For this review, take the finished solid that the model builds, in its own axes (mm). Face numbers are marked on the shaded views. A direction names the side the tool comes from. Give positions to 0.01 mm unless a question says otherwise; leave off trailing zeros. Loops run counter-clockwise (first coordinate to the right, second up) from the corner with the lowest first, then second, coordinate; pieces in that order, holes last. Notation, with made-up numbers: (37.5, 66) -> (71.5, 66) arc R20 ccw to (71.5, 85) -> close; hole circle Ø8 at (88, 13). An arc over 180 degrees is marked (long way). Answer as CSV lines item,"result". Start each with the question number.
Item 1: For L1, parallel to X at y = 6.75, z = -5.25; L2, parallel to Y at x = 1.25, z = -4.25, list the stretches that pass through material, from the lowest coordinate up. Write a range as from..to.
Item 2: The part is to be moulded in two halves that separate along Z. For the marked faces 1, 2 and 3, say which applies: +Z half, -Z half, draft (parallel to the pull), parting line (faces both ways), or undercut.
Item 3: Add section D-D on y = 10.25. State the section outline as (x, z) points, plus the area to 3 significant figures.
Item 4: Add section C-C on x = 1. State the section outline as (y, z) points, plus the area to 3 significant figures.
Item 5: Add section A-A on y = 2.75. State the section outline as (x, z) points.
Item 6: Clearance check with flat-ended pins moving along their axes: P1, Ø1, axis at x = -0.5, z = 2.5, coming from the +Y side; P2, Ø7.5, axis at x = -3.5, z = -2, coming from the +Y side. State where each tip first meets the part, or that it passes through.
Item 7: Machinability: for the marked faces 4 and 5, which of the approach directions +Z, -Z, +X, -X, +Y, -Y give a long, thin tool a straight path to every point of the face, cutting with its end or side? Answer none if there is none.
Item 8: Add section B-B on z = 1.5. State the section outline as (x, y) points, plus the area to 3 significant figures.
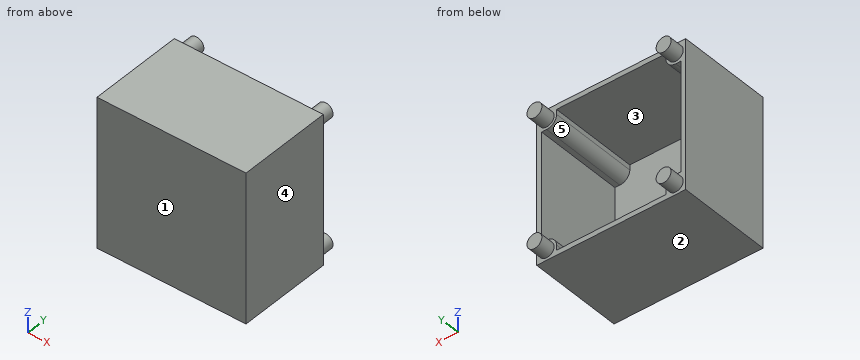
```python
from build123d import *

# Parameters (mm, degrees)
SKETCH_1_W          = 15
SKETCH_1_H          = 15
EXTRUDE_1_DEPTH     = 9.5
CUT_EXTRUDE_1_DEPTH = 9
SKETCH_5_R          = 0.75
EXTRUDE_2_DEPTH     = 1.5


with BuildPart() as part:
    # 草图1 → 凸台-拉伸1 (new body)
    with BuildSketch(Plane(origin=(0, 0, 0), x_dir=(1, 0, 0), z_dir=(0, 1, 0))):
        Rectangle(SKETCH_1_W, SKETCH_1_H)
    extrude(amount=EXTRUDE_1_DEPTH)

    # 草图2 → 切除-拉伸1 (cut)
    with BuildSketch(Plane(origin=(0, 9.5, 0), x_dir=(-1, 0, 0), z_dir=(0, 1, 0))):
        with BuildLine():
            Line((6.5, -5.5), (7, -5.5))
            Line((7, -5.5), (7, 5.5))
            Line((7, 5.5), (6.5, 5.5))
            ThreePointArc((6.5, 5.5), (5.792893219, 5.792893219), (5.5, 6.5))
            Line((5.5, 6.5), (5.5, 7))
            Line((5.5, 7), (-5.5, 7))
            Line((-5.5, 7), (-5.5, 6.5))
            ThreePointArc((-5.5, 6.5), (-5.792893219, 5.792893219), (-6.5, 5.5))
            Line((-6.5, 5.5), (-7, 5.5))
            Line((-7, 5.5), (-7, -5.5))
            Line((-7, -5.5), (-6.5, -5.5))
            ThreePointArc((-6.5, -5.5), (-5.792893219, -5.792893219), (-5.5, -6.5))
            Line((-5.5, -6.5), (-5.5, -7))
            Line((-5.5, -7), (5.5, -7))
            Line((5.5, -7), (5.5, -6.5))
            ThreePointArc((5.5, -6.5), (5.792893219, -5.792893219), (6.5, -5.5))
        make_face()
    extrude(amount=-CUT_EXTRUDE_1_DEPTH, mode=Mode.SUBTRACT)

    # 草图5 → 凸台-拉伸2 (add)
    with BuildSketch(Plane(origin=(0, 9.5, 0), x_dir=(-1, 0, 0), z_dir=(0, 1, 0))):
        with Locations(Location((6.5, -6.5, 0), (0, 0, 270))):
            Circle(SKETCH_5_R)
        with Locations(Location((6.5, 6.5, 0), (0, 0, 270))):
            Circle(SKETCH_5_R)
        with Locations(Location((-6.5, 6.5, 0), (0, 0, 270))):
            Circle(SKETCH_5_R)
        with Locations(Location((-6.5, -6.5, 0), (0, 0, 270))):
            Circle(SKETCH_5_R)
    extrude(amount=EXTRUDE_2_DEPTH)


solid = part.part
```
Computed values:
1,L1,"-7.5..-7, 7..7.5"
1,L2,"0..0.5"
2,face 1,"draft"
2,face 2,"-Z half"
2,face 3,"undercut"
3,outline,"circle Ø1.5 at (-6.5, -6.5); circle Ø1.5 at (-6.5, 6.5); circle Ø1.5 at (6.5, -6.5); circle Ø1.5 at (6.5, 6.5)"
3,area,"7.07 mm²"
4,outline,"(0, -7.5) -> (9.5, -7.5) -> (9.5, -7) -> (0.5, -7) -> (0.5, 7) -> (9.5, 7) -> (9.5, 7.5) -> (0, 7.5) -> close"
4,area,"16.5 mm²"
5,outline,"(-7.5, -7.5) -> (7.5, -7.5) -> (7.5, 7.5) -> (-7.5, 7.5) -> close; hole (-7, -5.5) -> (-6.5, -5.5) arc R1 cw to (-5.5, -6.5) -> (-5.5, -7) -> (5.5, -7) -> (5.5, -6.5) arc R1 cw to (6.5, -5.5) -> (7, -5.5) -> (7, 5.5) -> (6.5, 5.5) arc R1 cw to (5.5, 6.5) -> (5.5, 7) -> (-5.5, 7) -> (-5.5, 6.5) arc R1 cw to (-6.5, 5.5) -> (-7, 5.5) -> close"
6,P1,"y = 0.5"
6,P2,"y = 9.5"
7,face 4,"+Z, -Z, +X, +Y, -Y"
7,face 5,"+Y"
8,outline,"(-7.5, 0) -> (7.5, 0) -> (7.5, 9.5) -> (7, 9.5) -> (7, 0.5) -> (-7, 0.5) -> (-7, 9.5) -> (-7.5, 9.5) -> close"
8,area,"16.5 mm²"
